The listing builds one solid part. Answer for the finished solid, in the listing's coordinates (mm). Round coordinates to 2 decimals unless told otherwise and drop trailing zeros. Loops run counter-clockwise (first coordinate to the right, second up) from the corner with the lowest first, then second, coordinate; pieces in that order, holes last. Notation, with made-up numbers: (-23.75, 42) - (21.25, 42) arc R28 ccw to (21.25, 73) - close; hole circle Ø6 at (-7.75, 82). An arc over 180 degrees is marked (long way). One line per item, written item: value.
```python
from build123d import *

# Parameters (mm, degrees)
F1_DEPTH = 5.334


with BuildPart() as f1:
    # F0 (on Top) → F1 (new body)
    with BuildSketch(Plane.XY):
        with BuildLine():
            Line((-91.704233, 15.719872), (-110.754233, 15.719872))
            ThreePointArc((-110.754233, 15.719872), (-115.244361, 13.86), (-117.104233, 9.369872))
            Line((-117.104233, 9.369872), (-117.104233, -28.730128))
            ThreePointArc((-117.104233, -28.730128), (-115.244361, -33.220256), (-110.754233, -35.080128))
            Line((-110.754233, -35.080128), (35.295767, -35.080128))
            ThreePointArc((35.295767, -35.080128), (39.785895, -33.220256), (41.645767, -28.730128))
            Line((41.645767, -28.730128), (41.645767, 9.369872))
            ThreePointArc((41.645767, 9.369872), (39.785895, 13.86), (35.295767, 15.719872))
            Line((35.295767, 15.719872), (16.245767, 15.719872))
            Line((16.245767, 15.719872), (16.245767, -9.680128))
            Line((16.245767, -9.680128), (10.403767, -9.680128))
            Line((10.403767, -9.680128), (10.403767, 15.719872))
            Line((10.403767, 15.719872), (-85.862233, 15.719872))
            Line((-85.862233, 15.719872), (-85.862233, -9.680128))
            Line((-85.862233, -9.680128), (-91.704233, -9.680128))
            Line((-91.704233, -9.680128), (-91.704233, 15.719872))
        make_face()
    extrude(amount=F1_DEPTH)


solid = f1.part
```
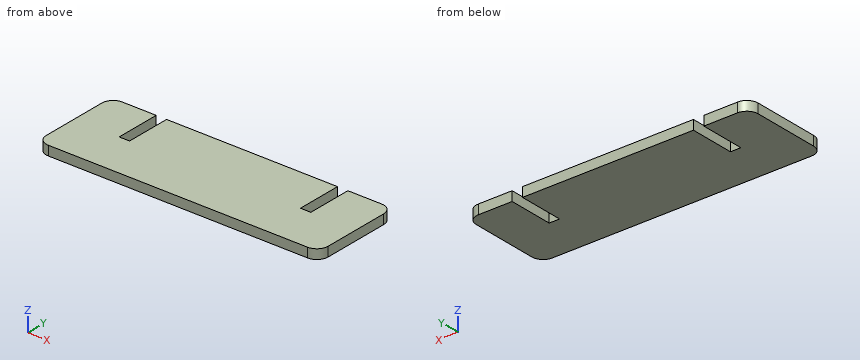
1) A cutting plane is placed at A-A on y = 4.5. Give the vertices of the cut face in (x, z).
Final values:
outline: (-117.1, 0) - (-91.7, 0) - (-91.7, 5.33) - (-117.1, 5.33) - close; (-85.86, 0) - (10.4, 0) - (10.4, 5.33) - (-85.86, 5.33) - close; (16.25, 0) - (41.65, 0) - (41.65, 5.33) - (16.25, 5.33) - close
2) This flat-tipped pin is pushed along its axis until it touches: pin 1 Ø1.6 at (x, z) = (-88, 3) entering from +Y. Where does it stop, or does it pass through?
Final values:
pin 1: y = -9.68
3) A cutting plane is placed at B-B on z = 2. Give the vertices of the cut face in (x, y), and give its area (3 significant figures).
Final values:
outline: (-117.1, -28.73) arc R6.35 ccw to (-110.75, -35.08) - (35.3, -35.08) arc R6.35 ccw to (41.65, -28.73) - (41.65, 9.37) arc R6.35 ccw to (35.3, 15.72) - (16.25, 15.72) - (16.25, -9.68) - (10.4, -9.68) - (10.4, 15.72) - (-85.86, 15.72) - (-85.86, -9.68) - (-91.7, -9.68) - (-91.7, 15.72) - (-110.75, 15.72) arc R6.35 ccw to (-117.1, 9.37) - close
area: 7,730 mm2
4) Consider L1, parallel to X at y = -9.5, z = 1.85; L2, parallel to Y at x = -89, z = 1.4; L3, parallel to X at y = 13, z = 3.4. Determine where each line is inside the solid, lowest interval first.
Final values:
L1: -117.1 to -91.7, -85.86 to 10.4, 16.25 to 41.65
L2: -35.08 to -9.68
L3: -115.96 to -91.7, -85.86 to 10.4, 16.25 to 40.51
